Could you check a few things on this drawing? It's one solid part, dimensions in mm from its lowest x, y, z. A direction names the side the tool comes from. Give positions to 0.01 mm unless a question says otherwise; leave off trailing zeros. Order: outer loops, then holes, each group sorted by start corner. A loop starts at its lowest first (then second) coordinate and runs counter-clockwise, first axis right, second up. Notation, with made-up numbers: (-34.5, 19) - (-23.5, 19) arc R15 cw to (-23.5, 24) - close; hole circle Ø4 at (39, 85). An arc over 180 degrees is marked (long way). Return JSON: item names as keys, results as strings.
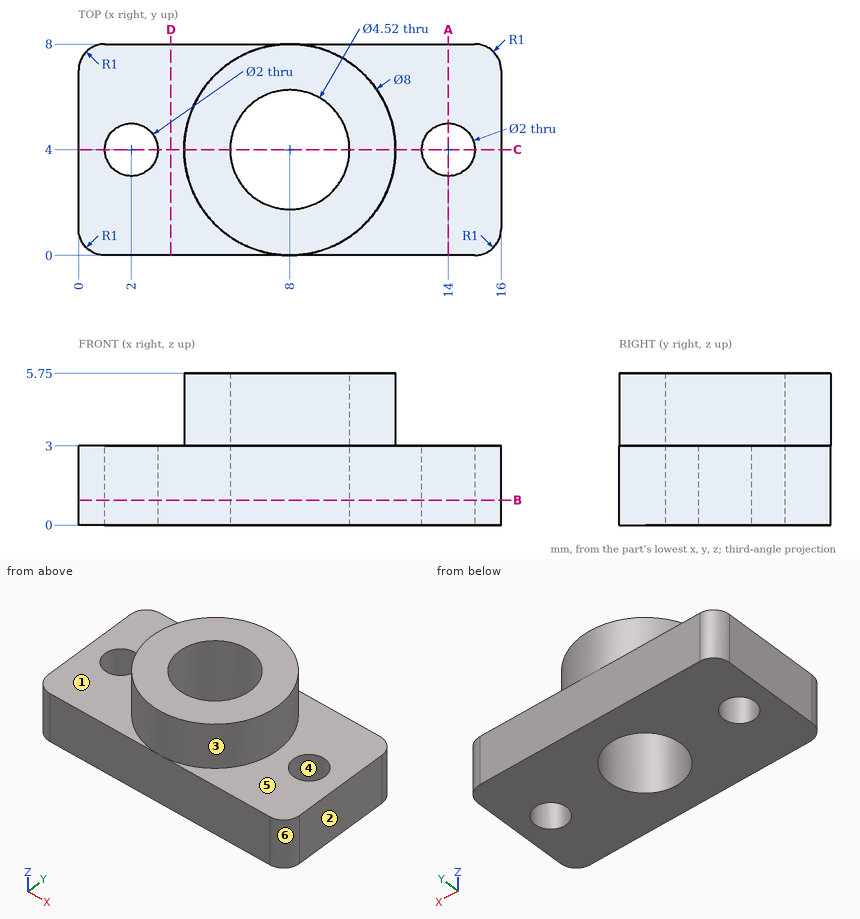
1. Suppose I cut it at A-A (x = 14). List the corners of the cut face in (y, z) for me.
Checks:
{"outline": "(0, 0) - (3, 0) - (3, 3) - (0, 3) - close; (5, 0) - (8, 0) - (8, 3) - (5, 3) - close"}
2. Thinking about a two-plate mould opening in X: for the marked faces 4, 5 and 6, which applies, +X half, -X half, draft (parallel to the pull), parting line (faces both ways), or undercut?
Checks:
{"face 4": "undercut", "face 5": "draft", "face 6": "+X half"}
3. If I drill on L1, parallel to Y at x = 2, z = 0.8; L2, parallel to X at y = 4.25, z = 1.35; L3, parallel to Y at x = 8, z = 3.3, over which ranges is the centre line in solid material (lowest first)? Write a range as [from, to].
Checks:
{"L1": "[0, 3], [5, 8]", "L2": "[0, 1.03], [2.97, 5.75], [10.25, 13.03], [14.97, 16]", "L3": "[0, 1.74], [6.26, 8]"}
4. Suppose I cut it at D-D (x = 3.5). List the corners of the cut face in (y, z) for me, plus the area to 3 significant figures.
Checks:
{"outline": "(0, 0) - (8, 0) - (8, 3) - (0, 3) - close", "area": "24.0 mm^2"}
5. On a 3-axis mill with a long thin cutter (end or side, diameter ignored), from which of +Z, -Z, +X, -X, +Y, -Y can I reach the whole of each face in a straight line? I mean the marked faces 1, 2 and 3. Say none if no direction works.
Checks:
{"face 1": "+Z, -X", "face 2": "+Z, -Z, +X, +Y, -Y", "face 3": "+Z"}
6. For pin 1 Ø1.8 at (x, y) = (2, 4) entering from -Z, with a flat end and sliding along its axis, tell me the tip position at first contact or that it passes through.
Checks:
{"pin 1": "through"}
7. Suppose I cut it at C-C (y = 4). List the corners of the cut face in (x, z) for me.
Checks:
{"outline": "(0, 0) - (1, 0) - (1, 3) - (0, 3) - close; (3, 0) - (5.74, 0) - (5.74, 5.75) - (4, 5.75) - (4, 3) - (3, 3) - close; (10.26, 0) - (13, 0) - (13, 3) - (12, 3) - (12, 5.75) - (10.26, 5.75) - close; (15, 0) - (16, 0) - (16, 3) - (15, 3) - close"}
8. Suppose I cut it at B-B (z = 0.95). List the corners of the cut face in (x, y) for me.
Checks:
{"outline": "(0, 1) arc R1 ccw to (1, 0) - (15, 0) arc R1 ccw to (16, 1) - (16, 7) arc R1 ccw to (15, 8) - (1, 8) arc R1 ccw to (0, 7) - close; hole circle Ø2 at (2, 4); hole circle Ø4.52 at (8, 4); hole circle Ø2 at (14, 4)"}
